from build123d import *

# Parameters (mm, degrees)
SCHIZZO1_W                        = 4
SCHIZZO1_H                        = 51.7
ESTRUSIONE_ESTRUSIONE1_DEPTH      = 1
SCHIZZO2_W                        = 1
SCHIZZO2_H                        = 4
ESTRUSIONE_ESTRUSIONE2_DEPTH      = 18
ESTRUSIONE_ESTRUSIONE2_DEPTH_BACK = 5.9
SCHIZZO3_W                        = 1
SCHIZZO3_H                        = 4
ESTRUSIONE_ESTRUSIONE3_DEPTH      = 18
ESTRUSIONE_ESTRUSIONE3_DEPTH_BACK = 5.9
SCHIZZO4_W                        = 4
SCHIZZO4_H                        = 1
ESTRUSIONE_ESTRUSIONE4_DEPTH      = 21.5
ESTRUSIONE_ESTRUSIONE4_DEPTH_BACK = 30.2
SCHIZZO5_W                        = 1
SCHIZZO5_H                        = 3
ESTRUSIONE_ESTRUSIONE5_DEPTH      = 21
SCHIZZO7_W                        = 1
SCHIZZO7_H                        = 4
ESTRUSIONE_ESTRUSIONE6_DEPTH      = 21
SCHIZZO8_W                        = 1
SCHIZZO8_H                        = 4
ESTRUSIONE_ESTRUSIONE7_DEPTH      = 21
SCHIZZO10_W                       = 4
SCHIZZO10_H                       = 1.3
ESTRUSIONE_ESTRUSIONE9_DEPTH      = 4.8
SCHIZZO11_W                       = 3.9
SCHIZZO11_H                       = 1.3
ESTRUSIONE_ESTRUSIONE10_DEPTH     = 4.8
SCHIZZO12_W                       = 1.2
SCHIZZO12_H                       = 1.2
ESTRUSIONE_ESTRUSIONE11_DEPTH     = 4
SCHIZZO13_W                       = 1
SCHIZZO13_H                       = 4
TAGLIO_ESTRUSIONE1_DEPTH          = 0.9
SCHIZZO14_W                       = 1
SCHIZZO14_H                       = 4
TAGLIO_ESTRUSIONE2_DEPTH          = 0.9
SCHIZZO15_W                       = 1
SCHIZZO15_H                       = 3
TAGLIO_ESTRUSIONE3_DEPTH          = 0.9
SCHIZZO16_W                       = 3.503631624
SCHIZZO16_H                       = 1
TAGLIO_ESTRUSIONE4_DEPTH          = 0.1
SCHIZZO17_W                       = 3.5
SCHIZZO17_H                       = 1
TAGLIO_ESTRUSIONE5_DEPTH          = 0.1
SCHIZZO18_W                       = 3.5
SCHIZZO18_H                       = 1
TAGLIO_ESTRUSIONE6_DEPTH          = 0.1
SCHIZZO19_W                       = 3.5
SCHIZZO19_H                       = 1
TAGLIO_ESTRUSIONE7_DEPTH          = 0.1
SCHIZZO20_W                       = 3.5
SCHIZZO20_H                       = 1
TAGLIO_ESTRUSIONE8_DEPTH          = 0.1
SCHIZZO21_W                       = 3.5
SCHIZZO21_H                       = 1
TAGLIO_ESTRUSIONE9_DEPTH          = 0.1
SCHIZZO22_W                       = 0.098173234
SCHIZZO22_H                       = 1.3
TAGLIO_ESTRUSIONE10_DEPTH         = 4.8


with BuildPart() as part:
    # Schizzo1 → Estrusione-Estrusione1 (new body)
    with BuildSketch(Plane.XY):
        with Locations((2, 25.85)):
            Rectangle(SCHIZZO1_W, SCHIZZO1_H)
    extrude(amount=ESTRUSIONE_ESTRUSIONE1_DEPTH)

    # Schizzo2 → Estrusione-Estrusione2 (add, two sides)
    with BuildSketch(Plane(origin=(4, 0, 0), x_dir=(0, 0, -1), z_dir=(1, 0, 0))) as estrusione_estrusione2_sk:
        with Locations((-0.5, 28.2)):
            Rectangle(SCHIZZO2_W, SCHIZZO2_H)
    extrude(amount=ESTRUSIONE_ESTRUSIONE2_DEPTH)
    extrude(estrusione_estrusione2_sk.sketch, amount=-ESTRUSIONE_ESTRUSIONE2_DEPTH_BACK)

    # Schizzo3 → Estrusione-Estrusione3 (add, two sides)
    with BuildSketch(Plane(origin=(4, 0, 0), x_dir=(0, 0, -1), z_dir=(1, 0, 0))) as estrusione_estrusione3_sk:
        with Locations((-0.5, 13)):
            Rectangle(SCHIZZO3_W, SCHIZZO3_H)
    extrude(amount=ESTRUSIONE_ESTRUSIONE3_DEPTH)
    extrude(estrusione_estrusione3_sk.sketch, amount=-ESTRUSIONE_ESTRUSIONE3_DEPTH_BACK)

    # Schizzo4 → Estrusione-Estrusione4 (add, two sides)
    with BuildSketch(Plane(origin=(0, 30.2, 0), x_dir=(1, 0, 0), z_dir=(0, 1, 0))) as estrusione_estrusione4_sk:
        with Locations((20, -0.5)):
            Rectangle(SCHIZZO4_W, SCHIZZO4_H)
    extrude(amount=ESTRUSIONE_ESTRUSIONE4_DEPTH)
    extrude(estrusione_estrusione4_sk.sketch, amount=-ESTRUSIONE_ESTRUSIONE4_DEPTH_BACK)

    # Schizzo5 → Estrusione-Estrusione5 (add)
    with BuildSketch(Plane(origin=(22, 0, 0), x_dir=(0, 0, -1), z_dir=(1, 0, 0))):
        with Locations((-0.5, 42.898738045)):
            Rectangle(SCHIZZO5_W, SCHIZZO5_H)
    extrude(amount=ESTRUSIONE_ESTRUSIONE5_DEPTH)

    # Schizzo7 → Estrusione-Estrusione6 (add)
    with BuildSketch(Plane(origin=(22, 0, 0), x_dir=(0, 0, -1), z_dir=(1, 0, 0))):
        with Locations((-0.5, 13)):
            Rectangle(SCHIZZO7_W, SCHIZZO7_H)
    extrude(amount=ESTRUSIONE_ESTRUSIONE6_DEPTH)

    # Schizzo8 → Estrusione-Estrusione7 (add)
    with BuildSketch(Plane(origin=(22, 0, 0), x_dir=(0, 0, -1), z_dir=(1, 0, 0))):
        with Locations((-0.5, 28.2)):
            Rectangle(SCHIZZO8_W, SCHIZZO8_H)
    extrude(amount=ESTRUSIONE_ESTRUSIONE7_DEPTH)

    # Schizzo10 → Estrusione-Estrusione9 (add)
    with BuildSketch(Plane(origin=(0, 0, 0), x_dir=(-1, 0, 0), z_dir=(0, 0, -1))):
        with Locations((-2, 42.81)):
            Rectangle(SCHIZZO10_W, SCHIZZO10_H)
    extrude(amount=ESTRUSIONE_ESTRUSIONE9_DEPTH)

    # Schizzo11 → Estrusione-Estrusione10 (add)
    with BuildSketch(Plane(origin=(0, 0, 0), x_dir=(-1, 0, 0), z_dir=(0, 0, -1))):
        with Locations((-19.95, 42.91)):
            Rectangle(SCHIZZO11_W, SCHIZZO11_H)
    extrude(amount=ESTRUSIONE_ESTRUSIONE10_DEPTH)

    # Schizzo12 → Estrusione-Estrusione11 (add)
    with BuildSketch(Plane(origin=(0, 0, 0), x_dir=(-1, 0, 0), z_dir=(0, 0, -1))):
        with Locations((-40.765421969, 42.965995875)):
            Rectangle(SCHIZZO12_W, SCHIZZO12_H)
    extrude(amount=ESTRUSIONE_ESTRUSIONE11_DEPTH)

    # Schizzo13 → Taglio-Estrusione1 (cut)
    with BuildSketch(Plane(origin=(43, 0, 0), x_dir=(0, 0, -1), z_dir=(1, 0, 0))):
        with Locations((-0.5, 28.2)):
            Rectangle(SCHIZZO13_W, SCHIZZO13_H)
    extrude(amount=-TAGLIO_ESTRUSIONE1_DEPTH, mode=Mode.SUBTRACT)

    # Schizzo14 → Taglio-Estrusione2 (cut)
    with BuildSketch(Plane(origin=(43, 0, 0), x_dir=(0, 0, -1), z_dir=(1, 0, 0))):
        with Locations((-0.5, 13)):
            Rectangle(SCHIZZO14_W, SCHIZZO14_H)
    extrude(amount=-TAGLIO_ESTRUSIONE2_DEPTH, mode=Mode.SUBTRACT)

    # Schizzo15 → Taglio-Estrusione3 (cut)
    with BuildSketch(Plane(origin=(43, 0, 0), x_dir=(0, 0, -1), z_dir=(1, 0, 0))):
        with Locations((-0.5, 42.898738045)):
            Rectangle(SCHIZZO15_W, SCHIZZO15_H)
    extrude(amount=-TAGLIO_ESTRUSIONE3_DEPTH, mode=Mode.SUBTRACT)

    # Schizzo16 → Taglio-Estrusione4 (cut)
    with BuildSketch(Plane.XZ.offset(-11)):
        with Locations((40.348184188, 0.5)):
            Rectangle(SCHIZZO16_W, SCHIZZO16_H)
    extrude(amount=-TAGLIO_ESTRUSIONE4_DEPTH, mode=Mode.SUBTRACT)

    # Schizzo17 → Taglio-Estrusione5 (cut)
    with BuildSketch(Plane(origin=(0, 15, 0), x_dir=(1, 0, 0), z_dir=(0, 1, 0))):
        with Locations((40.35, -0.5)):
            Rectangle(SCHIZZO17_W, SCHIZZO17_H)
    extrude(amount=-TAGLIO_ESTRUSIONE5_DEPTH, mode=Mode.SUBTRACT)

    # Schizzo18 → Taglio-Estrusione6 (cut)
    with BuildSketch(Plane(origin=(0, 30.2, 0), x_dir=(1, 0, 0), z_dir=(0, 1, 0))):
        with Locations((40.35, -0.5)):
            Rectangle(SCHIZZO18_W, SCHIZZO18_H)
    extrude(amount=-TAGLIO_ESTRUSIONE6_DEPTH, mode=Mode.SUBTRACT)

    # Schizzo19 → Taglio-Estrusione7 (cut)
    with BuildSketch(Plane(origin=(0, 26.2, 0), x_dir=(-1, 0, 0), z_dir=(0, -1, 0))):
        with Locations((-40.35, -0.5)):
            Rectangle(SCHIZZO19_W, SCHIZZO19_H)
    extrude(amount=-TAGLIO_ESTRUSIONE7_DEPTH, mode=Mode.SUBTRACT)

    # Schizzo20 → Taglio-Estrusione8 (cut)
    with BuildSketch(Plane(origin=(0, 41.398738045, 0), x_dir=(-1, 0, 0), z_dir=(0, -1, 0))):
        with Locations((-40.35, -0.5)):
            Rectangle(SCHIZZO20_W, SCHIZZO20_H)
    extrude(amount=-TAGLIO_ESTRUSIONE8_DEPTH, mode=Mode.SUBTRACT)

    # Schizzo21 → Taglio-Estrusione9 (cut)
    with BuildSketch(Plane(origin=(0, 44.398738045, 0), x_dir=(1, 0, 0), z_dir=(0, 1, 0))):
        with Locations((40.35, -0.5)):
            Rectangle(SCHIZZO21_W, SCHIZZO21_H)
    extrude(amount=-TAGLIO_ESTRUSIONE9_DEPTH, mode=Mode.SUBTRACT)

    # Schizzo22 → Taglio-Estrusione10 (cut)
    with BuildSketch(Plane(origin=(0, 0, -4.8), x_dir=(-1, 0, 0), z_dir=(0, 0, -1))):
        with Locations((-18.049086617, 42.91)):
            Rectangle(SCHIZZO22_W, SCHIZZO22_H)
    extrude(amount=-TAGLIO_ESTRUSIONE10_DEPTH, mode=Mode.SUBTRACT)


solid = part.part
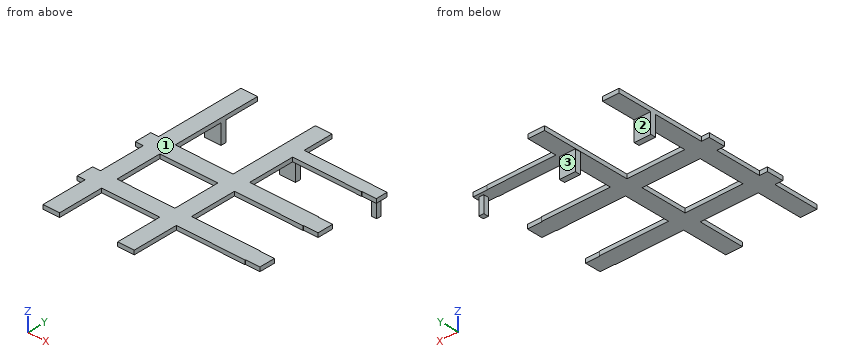
Can you work these out from the model? Positions are in its coordinate system, mm. Face numbers are marked on the shaded views. A direction names the side the tool comes from. Round coordinates to 2 decimals unless told otherwise and drop trailing zeros. Write each loop counter-clockwise with the first axis right and the second up, starting at its lowest first coordinate (ties: lowest second). Pieces come first, ordered by that corner, then holes. Notation, with made-up numbers: M 58.5,-1 L 63.5,-1 A35 ccw 63.5,37 Z; hole C -39,26 d1. An arc over 180 degrees is marked long. Use a Markdown table: item, result.
Item 1: I want a section at A-A (y = 9). List the corners of the cut face in (x, z) for me.
Found:
| item | result |
|---|---|
| outline | M 0,0 L 4,0 L 4,1 L 0,1 Z; M 18,0 L 22,0 L 22,1 L 18,1 Z |
Item 2: I want a section at D-D (x = 17). List the corners of the cut face in (y, z) for me.
Found:
| item | result |
|---|---|
| outline | M 11,0 L 15,0 L 15,1 L 11,1 Z; M 26.2,0 L 30.2,0 L 30.2,1 L 26.2,1 Z |
Item 3: Which directions (+Z, -Z, +X, -X, +Y, -Y) give clear straight access to the entire face, cutting with the end or side of a thin tool? Please do the marked faces 1, 2 and 3.
Found:
| item | result |
|---|---|
| face 1 | +Z, +X, -X, +Y, -Y |
| face 2 | -Z, -X, +Y |
| face 3 | -Z, +X, -X, +Y |
Item 4: For pin 1 Ø1.1 at (x, z) = (8, 0.5) entering from +Y; pin 2 Ø0.5 at (x, z) = (13, 0.5) entering from -Y; pin 3 Ø0.8 at (x, z) = (40, 0.5) entering from -Y, each with a flat end and sliding along its axis, tell me the tip position at first contact or that it passes through.
Found:
| item | result |
|---|---|
| pin 1 | stops at y = 30.2 |
| pin 2 | stops at y = 11 |
| pin 3 | stops at y = 11.1 |
Item 5: I want a section at C-C (z = -1.1). List the corners of the cut face in (x, y) for me, and give its area (3 significant figures).
Found:
| item | result |
|---|---|
| outline | M 0,42.16 L 4,42.16 L 4,43.46 L 0,43.46 Z; M 18.1,42.26 L 21.9,42.26 L 21.9,43.56 L 18.1,43.56 Z; M 40.17,42.37 L 41.37,42.37 L 41.37,43.57 L 40.17,43.57 Z |
| area | 11.6 mm2 |
Item 6: I want a section at B-B (x = 24). List the corners of the cut face in (y, z) for me, and give its area (3 significant figures).
Found:
| item | result |
|---|---|
| outline | M 11,0 L 15,0 L 15,1 L 11,1 Z; M 26.2,0 L 30.2,0 L 30.2,1 L 26.2,1 Z; M 41.4,0 L 44.4,0 L 44.4,1 L 41.4,1 Z |
| area | 11.0 mm2 |
Item 7: If I drill on line 1 along Y through (x, z) = (25, 0.6); line 2 along Z through (x, y) = (24, 27); line 3 along Y through (x, z) = (19, -0.7), over which ranges is the centre line in solid material (lowest first)? Write a range as [from, to].
Found:
| item | result |
|---|---|
| line 1 | y = [11, 15], [26.2, 30.2], [41.4, 44.4] |
| line 2 | z = [0, 1] |
| line 3 | y = [42.26, 43.56] |
